Check sheet for the modelled part. Datum: model origin and axes. Units: mm. A direction names the side the tool comes from. Coordinates: 2 decimals unless noted, no trailing zeros. Loops run counter-clockwise (first coordinate to the right, second up) from the corner with the lowest first, then second, coordinate; pieces in that order, holes last. Notation, with made-up numbers: M -28.5,50 L -5.5,50 A16 ccw -5.5,57 Z; hole C -11.75,64.5 d4. An arc over 180 degrees is marked long. Answer in a Markdown table with one row per item. Add a question column.
```python
from build123d import *

# Parameters (mm, degrees)
SKETCH2_W           = 100
SKETCH2_H           = 40
BOSS_EXTRUDE1_DEPTH = 10
SKETCH4_W           = 100
SKETCH4_H           = 15
BOSS_EXTRUDE2_DEPTH = 63.33333
FILLET1_R           = 25
FILLET2_R           = 25
SKETCH5_W           = 100
SKETCH5_H           = 15
BOSS_EXTRUDE3_DEPTH = 5
FILLET3_R           = 25
FILLET4_R           = 25
FILLET10_R          = 10
FILLET11_R          = 10


with BuildPart() as part:
    # Sketch2 → Boss-Extrude1 (new body)
    with BuildSketch(Plane(origin=(0, 0, 0), x_dir=(1, 0, 0), z_dir=(0, 1, 0))):
        Rectangle(SKETCH2_W, SKETCH2_H)
    extrude(amount=BOSS_EXTRUDE1_DEPTH)

    # Sketch4 → Boss-Extrude2 (add)
    with BuildSketch(Plane(origin=(0, 0, 0), x_dir=(1, 0, 0), z_dir=(0, 1, 0))):
        with Locations((0, -12.5)):
            Rectangle(SKETCH4_W, SKETCH4_H)
        with Locations((0, 12.5)):
            Rectangle(SKETCH4_W, SKETCH4_H)
    extrude(amount=BOSS_EXTRUDE2_DEPTH)

    # Fillet1
    # the kernel refuses this fillet: 25 mm, written as the material it takes off along each edge
    with BuildSketch(Plane(origin=(107.282196187, 63.33333, 5), x_dir=(0, 0, 1), z_dir=(-1, 0, 0))) as fillet1_piece_1:
        with BuildLine():
            CenterArc((25, -22.912878475), FILLET1_R, 113.578178478, 66.421821522)
            Line((0, -22.912878475), (-0.5, -22.912878475))
            Line((-0.5, -22.912878475), (-0.5, 0))
            Line((-0.5, 0), (0, 0.5))
            ThreePointArc((0, 0.5), (7.5, 0.5), (14.8, 0.458257569))
            Line((14.8, 0.458257569), (15, 0))
        make_face()
    extrude(amount=214.564392374, mode=Mode.SUBTRACT)

    # Fillet2
    # the kernel refuses this fillet: 25 mm, written as the material it takes off along each edge
    with BuildSketch(Plane(origin=(107.282196187, 63.33333, -5), x_dir=(0, 0, -1), z_dir=(-1, 0, 0))) as fillet2_piece_1:
        with BuildLine():
            CenterArc((25, 22.912878475), FILLET2_R, 180, 66.421821522)
            Line((0, 22.912878475), (-0.5, 22.912878475))
            Line((-0.5, 22.912878475), (-0.5, 0))
            Line((-0.5, 0), (0, -0.5))
            ThreePointArc((0, -0.5), (7.5, -0.5), (14.8, -0.458257569))
            Line((14.8, -0.458257569), (15, 0))
        make_face()
    extrude(amount=214.564392374, mode=Mode.SUBTRACT)

    # Sketch5 → Boss-Extrude3 (add)
    with BuildSketch(Plane(origin=(0, 0, 0), x_dir=(1, 0, 0), z_dir=(0, 1, 0))):
        with Locations((0, -27.5)):
            Rectangle(SKETCH5_W, SKETCH5_H)
        with Locations((0, 27.5)):
            Rectangle(SKETCH5_W, SKETCH5_H)
    extrude(amount=BOSS_EXTRUDE3_DEPTH)

    # Fillet3
    # the kernel refuses this fillet: 25 mm, written as the material it adds along each edge
    with BuildSketch(Plane(origin=(-50, 5, 20), x_dir=(0, 1, 0), z_dir=(1, 0, 0))) as fillet3_piece_1:
        with BuildLine():
            CenterArc((22.912878475, 25), FILLET3_R, 203.578178478, 66.421821522)
            Line((0, 15), (-0.458257569, 14.8))
            ThreePointArc((-0.458257569, 14.8), (-0.5, 7.5), (-0.5, 0))
            Line((-0.5, 0), (0, -0.5))
            Line((0, -0.5), (22.912878475, -0.5))
            Line((22.912878475, -0.5), (22.912878475, 0))
        make_face()
    extrude(amount=100)

    # Fillet4
    # the kernel refuses this fillet: 25 mm, written as the material it adds along each edge
    with BuildSketch(Plane(origin=(-50, 5, -20), x_dir=(0, 1, 0), z_dir=(1, 0, 0))) as fillet4_piece_1:
        with BuildLine():
            CenterArc((22.912878475, -25), FILLET4_R, 90, 66.421821522)
            Line((0, -15), (-0.458257569, -14.8))
            ThreePointArc((-0.458257569, -14.8), (-0.5, -7.5), (-0.5, 0))
            Line((-0.5, 0), (0, 0.5))
            Line((0, 0.5), (22.912878475, 0.5))
            Line((22.912878475, 0.5), (22.912878475, 0))
        make_face()
    extrude(amount=100)

    # Fillet10
    fillet10_edges = [part.edges().sort_by_distance(p)[0] for p in [
        (-50, 14.219814537, -24.083499337),
        (-50, 45.623104237, -20),
    ]]
    fillet(fillet10_edges, radius=FILLET10_R)

    # Fillet11
    fillet11_edges = [part.edges().sort_by_distance(p)[0] for p in [
        (50, 14.219814537, -24.083499337),
        (50, 14.219814537, 24.083499337),
        (-50, 14.219814537, 24.083499337),
        (50, 45.623104237, -20),
        (50, 45.623104237, 20),
        (-50, 45.623104237, 20),
    ]]
    fillet(fillet11_edges, radius=FILLET11_R)


solid = part.part
```
Q1. Mould release check, pull along Z, two halves, no side actions. Record for faces 1 (the face through (50, 17.6, 5.4)), 2 (the face through (-0.56, 14.051, 24.195)), 3 (the face through (-0.56, 14.39, -23.973)), 4 (the face through (-1, 10, 0)): released by +Z, released by -Z, zero draft, split by the parting line, or undercut.
Q2. Cross-section at A-A (y = 37). Record the cut outline in (x, z), plus the area to 3 significant figures.
Q3. Thickness scan on L1, parallel to Z at x = 40.5, y = 32; L2, parallel to Z at x = -32.5, y = 12; L3, parallel to Y at x = -15.5, z = -10. Record the ranges inside material, lowest first.
Q4. Go/stop test with flat-tipped pins: pin 1 (1 mm diameter, centred on x = 28.5, y = 38, fed in from +Z); pin 2 (24.5 mm diameter, centred on x = 23, y = 21.5, fed in from -Z); pin 3 (8 mm diameter, centred on x = 33.5, y = 17.5, fed in from -Z). Record where each tip stops, or that it passes through.
Q5. Cross-section at B-B (x = 27.5). Record the cut outline in (y, z), plus the area to 3 significant figures.
Q6. Cross-section at C-C (y = 58). Record the cut outline in (x, z), plus the area to 3 significant figures.
Q7. Cross-section at D-D (z = -7). Record the cut outline in (x, y), plus the area to 3 significant figures.
Q8. Access from +Z, -Z, +X, -X, +Y, -Y to the whole of each face (thin tool, end or side, straight path). Record for faces 5 (the face through (-1, 25, -5)), 6 (the face through (-1, 45, 20)), 7 (the face through (-46.99, 45.38, -17.15)), 8 (the face through (46.99, 45.38, -17.15)).
Answer key:
| question | item | result |
|---|---|---|
| 1 | face 1 | zero draft |
| 1 | face 2 | released by +Z |
| 1 | face 3 | released by -Z |
| 1 | face 4 | undercut |
| 2 | outline | M -50,-10 A10 ccw -40,-20 L 40,-20 A10 ccw 50,-10 L 50,-5 L -50,-5 Z; M -50,5 L 50,5 L 50,10 A10 ccw 40,20 L -40,20 A10 ccw -50,10 Z |
| 2 | area | 2,910 mm^2 |
| 3 | L1 | -19.99 to -5, 5 to 19.99 |
| 3 | L2 | -25.72 to -5, 5 to 25.72 |
| 3 | L3 | 0 to 55.42 |
| 4 | pin 1 | z = 20 |
| 4 | pin 2 | z = -28.37 |
| 4 | pin 3 | z = -24.57 |
| 5 | outline | M 0,-35 L 5,-35 A25 cw 27.91,-20 L 63.33,-20 A25 ccw 40.42,-5 L 10,-5 L 10,5 L 40.42,5 A25 ccw 63.33,20 L 27.91,20 A25 cw 5,35 L 0,35 Z |
| 5 | area | 2,150 mm^2 |
| 6 | outline | M -49.75,-12.22 A10 ccw -40,-20 L 40,-20 A10 ccw 49.75,-12.22 Z; M -49.75,12.22 L 49.75,12.22 A10 ccw 40,20 L -40,20 A10 ccw Z |
| 6 | area | 1,470 mm^2 |
| 7 | outline | M -50,0 L 50,0 L 50,50.22 L -50,50.22 Z |
| 7 | area | 5,020 mm^2 |
| 8 | face 5 | +X, -X, +Y |
| 8 | face 6 | +Z, +X, -X, +Y |
| 8 | face 7 | -Z, -X, +Y |
| 8 | face 8 | -Z, +X, +Y |
